from build123d import *

# Parameters (mm, degrees)
SKETCH1_R           = 8
BOSS_EXTRUDE1_DEPTH = 1
SKETCH2_R           = 6.75
BOSS_EXTRUDE2_DEPTH = 5
SKETCH3_R           = 2
CUT_EXTRUDE1_DEPTH  = 13.806248475
CUT_EXTRUDE1_DRAFT  = -1


with BuildPart() as part:
    # Sketch1 → Boss-Extrude1 (new body)
    with BuildSketch(Plane(origin=(0, 0, 0), x_dir=(1, 0, 0), z_dir=(0, 1, 0))):
        with Locations(Location((0, 0, 0), (0, 0, 270))):
            Circle(SKETCH1_R)
    extrude(amount=BOSS_EXTRUDE1_DEPTH)

    # Sketch2 → Boss-Extrude2 (add)
    with BuildSketch(Plane(origin=(0, 1, 0), x_dir=(1, 0, 0), z_dir=(0, 1, 0))):
        with Locations(Location((0, 0, 0), (0, 0, 270))):
            Circle(SKETCH2_R)
    extrude(amount=BOSS_EXTRUDE2_DEPTH)


with BuildPart() as cut_extrude1_tool:
    # Sketch3 → Cut-Extrude1 (with draft: the straight prism first)
    with BuildSketch(Plane.XZ):
        Circle(SKETCH3_R)
    extrude(amount=-CUT_EXTRUDE1_DEPTH)
    # Cut-Extrude1: the draft: its side faces are tilted about the plane it starts from
    cut_extrude1_sides = [cut_extrude1_tool.faces().sort_by_distance(p)[0] for p in [
        (-2, 6.903124237, 0),
    ]]
    draft(cut_extrude1_sides, Plane.XZ, CUT_EXTRUDE1_DRAFT)


with BuildPart() as part_1:
    add(part.part)

    # Cut-Extrude1: cut by cut_extrude1_tool
    add(cut_extrude1_tool.part, mode=Mode.SUBTRACT)


solid = part_1.part
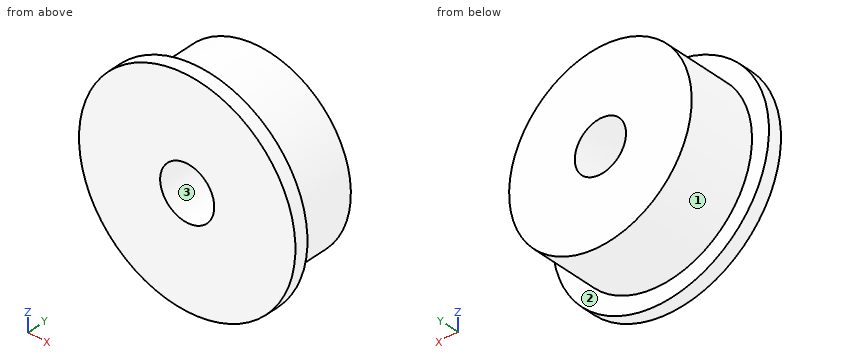
Geometry: final body of the model. Coordinates: model frame, mm. Face numbers are marked on the shaded views. Coordinates: 2 decimals unless noted, no trailing zeros. Order: outer loops, then holes, each group sorted by start corner. A loop starts at its lowest first (then second) coordinate and runs counter-clockwise, first axis right, second up.
1) Draft query along Z for the marked faces 1, 2 and 3. Return one class per face: released by +Z, released by -Z, zero draft, split by the parting line, or undercut.
Result sheet:
face 1: split by the parting line
face 2: zero draft
face 3: undercut
2) Section D-D (y = 5.75). Return loops of the section in (x, z).
Result sheet:
outline: circle Ø13.5 at (0, 0); hole circle Ø3.8 at (0, 0)
3) Section C-C (y = 3). Return loops of the section in (x, z).
Result sheet:
outline: circle Ø13.5 at (0, 0); hole circle Ø3.9 at (0, 0)
4) Section A-A (x = 5.75). Return loops of the section in (y, z), then the cut area to 3 significant figures.
Result sheet:
outline: (0, -5.56) - (1, -5.56) - (1, -3.54) - (6, -3.54) - (6, 3.54) - (1, 3.54) - (1, 5.56) - (0, 5.56) - close
area: 46.5 mm2
5) Section B-B (z = -3.75). Return loops of the section in (x, y), then the cut area to 3 significant figures.
Result sheet:
outline: (-7.07, 0) - (7.07, 0) - (7.07, 1) - (5.61, 1) - (5.61, 6) - (-5.61, 6) - (-5.61, 1) - (-7.07, 1) - close
area: 70.3 mm2
6) Ray query, probe 1 along Y at (x, z) = (-3.5, -6.5); probe 2 along Z at (x, y) = (1.75, 5); probe 3 along X at (y, z) = (2.5, 0.25). Return the intervals inside material, ascending.
Result sheet:
probe 1: y = 0 to 1
probe 2: z = -6.52 to -0.77, 0.77 to 6.52
probe 3: x = -6.75 to -1.94, 1.94 to 6.75
7) First-contact query: P1, Ø1.5, axis at y = 1.5, z = 1.5, coming from the -X side; P2, Ø1.5, axis at y = 2, z = 1, coming from the -X side; P3, Ø6, axis at x = -0.5, z = 4.5, coming from the -Y side. Flat tips, straight axial feed; report the tip coordinate or a pass-through.
Result sheet:
P1: stops at x = -7.94
P2: stops at x = -6.75
P3: stops at y = 0
